```python
from build123d import *

# Parameters (mm, degrees)
F0_R     = 38.1
F1_DEPTH = 12.7
F2_R     = 63.5
F2_R_2   = 38.1
F3_DEPTH = 34.925
F4_SIZE  = 6.35


with BuildPart() as f1:
    # F0 (on Right) → F1 (new body, symmetric)
    with BuildSketch(Plane.YZ):
        with BuildLine():
            ThreePointArc((139.12153, 88.9), (165.1, 0), (139.12153, -88.9))
            Line((139.12153, -88.9), (338.394032, -62.969102))
            ThreePointArc((338.394032, -62.969102), (393.7, 0), (338.394032, 62.969102))
            Line((338.394032, 62.969102), (139.12153, 88.9))
        make_face()
        with Locations((330.2, 0)):
            Circle(F0_R, mode=Mode.SUBTRACT)
    extrude(amount=F1_DEPTH, both=True)

    # F2 (on Right) → F3 (join, symmetric)
    with BuildSketch(Plane.YZ):
        with Locations((330.2, 0)):
            Circle(F2_R)
        with Locations((330.2, 0)):
            Circle(F2_R_2, mode=Mode.SUBTRACT)
    extrude(amount=F3_DEPTH, both=True)

    # F4
    f4_edges = [f1.edges().sort_by_distance(p)[0] for p in [
        (-34.925, 292.1, 0),
        (34.925, 292.1, 0),
    ]]
    chamfer(f4_edges, length=F4_SIZE)


solid = f1.part
```
Geometry check sheet. Reference: the model listing, model coordinates, mm. Round coordinates to 2 decimals unless told otherwise and drop trailing zeros. Order: outer loops, then holes, each group sorted by start corner. A loop starts at its lowest first (then second) coordinate and runs counter-clockwise, first axis right, second up. Notation, with made-up numbers: (64.25, -36) - (97.25, -36) arc R23 cw to (97.25, -25) - close; hole circle Ø5 at (-20, -8.75). An arc over 180 degrees is marked (long way). Use a Markdown table: item, result. Add a question column.
(1) Material ranges on line 1 along Z through (x, y) = (13, 330.2); line 2 along X through (y, z) = (164, -56); line 3 along Y through (x, z) = (-10.5, 24.5), recorded low to high. Write a range as [from, to].
(2) Depth check by flat-ended pin: pin 1 (8 mm diameter, centred on x = -26.5, y = 277, fed in from -Z); pin 2 (8 mm diameter, centred on x = 7, y = 200, fed in from -Z); pin 3 (1.5 mm diameter, centred on x = 12.5, y = 276.5, fed in from -Z). Enter the tip coordinate at first touch or a pass-through.
(3) Release check for a two-part mould opening along Z. For faces 1 (the flat face through (12.7, 215, 1)), 2 (the flat face through (0.178, 240.153, 75.753)), 3 (the cylindrical face through (0.178, 165.095, 1.314)) record: pulls with the +Z half, pulls with the -Z half, needs draft (parallel to the pull), parting line crosses it, or undercut.
(4) Sectioned sample at A-A, the plane z = 0. Enter the section's corners in (x, y) (3 decimals).
(5) Sectioned sample at D-D, the plane z = -58.5. Enter the section's corners in (x, y) (3 decimals).
(6) Sectioned sample at B-B, the plane x = -4.5. Enter the section's corners in (y, z), and give its area (3 significant figures).
(7) Sectioned sample at C-C, the plane y = 330.2. Enter the section's corners in (x, z) (3 decimals).
Answers below:
| question | item | result |
|---|---|---|
| 1 | line 1 | [-63.5, -38.1], [38.1, 63.5] |
| 1 | line 2 | [-12.7, 12.7] |
| 1 | line 3 | [163.27, 301.02], [359.38, 388.78] |
| 2 | pin 1 | z = -40.14 |
| 2 | pin 2 | z = -81.5 |
| 2 | pin 3 | z = -71.12 |
| 3 | face 1 | needs draft |
| 3 | face 2 | pulls with the +Z half |
| 3 | face 3 | undercut |
| 4 | outline | (-34.925, 266.7) - (-12.7, 266.7) - (-12.7, 165.1) - (12.7, 165.1) - (12.7, 266.7) - (34.925, 266.7) - (34.925, 285.75) - (28.575, 292.1) - (-28.575, 292.1) - (-34.925, 285.75) - close; (-34.925, 374.65) - (-28.575, 368.3) - (28.575, 368.3) - (34.925, 374.65) - (34.925, 393.7) - (-34.925, 393.7) - close |
| 5 | outline | (-34.925, 305.502) - (-12.7, 305.502) - (-12.7, 154.388) - (12.7, 154.388) - (12.7, 305.502) - (34.925, 305.502) - (34.925, 354.898) - (-34.925, 354.898) - close |
| 6 | outline | (139.12, -88.9) - (338.39, -62.97) arc R63.5 ccw to (338.39, 62.97) - (139.12, 88.9) arc R165.1 cw to start; hole circle Ø76.2 at (330.2, 0) |
| 6 | area | 27,900 mm² |
| 7 | outline | (-34.925, -63.5) - (-12.7, -63.5) - (-12.7, -64.035) - (12.7, -64.035) - (12.7, -63.5) - (34.925, -63.5) - (34.925, -44.45) - (28.575, -38.1) - (-28.575, -38.1) - (-34.925, -44.45) - close; (-34.925, 44.45) - (-28.575, 38.1) - (28.575, 38.1) - (34.925, 44.45) - (34.925, 63.5) - (12.7, 63.5) - (12.7, 64.035) - (-12.7, 64.035) - (-12.7, 63.5) - (-34.925, 63.5) - close |
